Input: part model. Units: mm. Frame: model coordinates. Coordinates: 2 decimals unless noted, no trailing zeros. Loops run counter-clockwise (first coordinate to the right, second up) from the corner with the lowest first, then second, coordinate; pieces in that order, holes last.
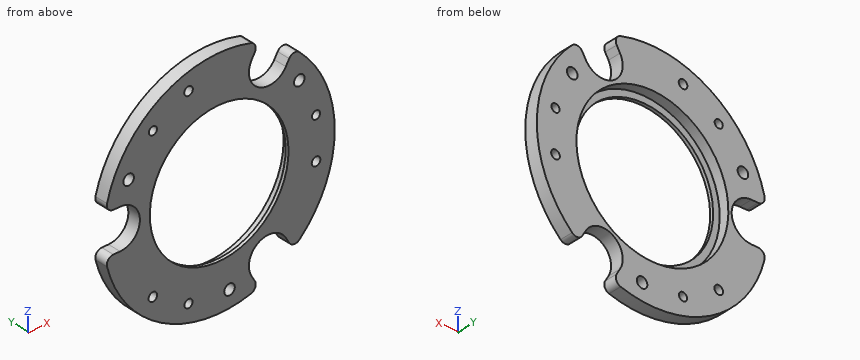
Autodesk Inventor part; units mm, degrees
ref_plane "YZ Plane" through (0, 0, 0) normal (1, 0, 0) x (0, 1, 0)
ref_plane "XZ Plane" through (0, 0, 0) normal (0, 1, 0) x (-1, 0, 0)
ref_plane "XY Plane" through (0, 0, 0) normal (0, 0, 1) x (1, 0, 0)
sketch "Sketch1" plane through (0, 0, 0) normal (1, 0, 0) x (0, 1, 0)
  line L0 (0, 35) -> (4, 35)
  line L1 (4, 35) -> (4, 23)
  line L2 (1, 21) -> (0, 21)
  line L3 (0, 21) -> (0, 35)
  line L4 (-0.8, 0) -> (4.8, 0)
  line L5 (1, 23) -> (1, 21)
  line L6 (4, 23) -> (1, 23)
  point P0 (0, 0)
  dimension "d0" = 21
  dimension "d2" = 35
  dimension "d51" = 4
  dimension "d52" = 3
  dimension "d53" = 23
revolve "Revolution1" add sketch "Sketch1" angle 360 about axis through (0, -10, 0) along (0, 1, 0)
sketch "Sketch2" plane through (0, 4, 0) normal (0, 1, 0) x (1, 0, 0)
  arc A0 (-30, -6) -> (-30, 6) centre (-30, 0) ccw
  line L0 (-30, -6) -> (-34.4819, -6)
  circle A1 centre (0, 0) radius 35
  line L1 (-30, 6) -> (-34.4819, 6)
  arc A2 (-34.4819, 6) -> (-34.4819, -6) centre (0, 0) ccw
  dimension "d6" = 12
  dimension "d7" = 30
extrude "Extrusion1" cut sketch "Sketch2" against normal blind 4 contours L0 A1 L1 A0 picked at (-31.3095, 0.2411)
pattern_circular "Circular Pattern1" count 3 over 360 about axis through (0, 0.5, 0) along (0, 1, 0) of "Extrusion1"
sketch "Sketch3" plane through (-34.4819, 4, -6) normal (0, 1, 0) x (1, 0, 0)
  point P0 (34.4819, -6)
sketch "Sketch4" plane through (-34.4819, 4, -6) normal (0, 1, 0) x (1, 0, 0)
  circle A0 centre (34.4819, -6) radius 30 construction
  arc A1 (4.4819, -12) -> (4.4819, 0) centre (4.4819, -6) ccw
  point P0 (7.0755, -18.2021)
  dimension "d13" = 60
  dimension "d14" = 24
hole "Hole1" at (-27.4064, 4, 12.2021) direction (0, -1, 0) diameter 3.2 end through all
pattern_circular "Circular Pattern2" count 3 over 360 about axis through (0, 0.5, 0) along (0, 1, 0) of "Hole1"
sketch "Sketch5" plane through (-34.4819, 4, -6) normal (0, 1, 0) x (1, 0, 0)
  circle A0 centre (34.4819, -6) radius 30 construction
  arc A1 (4.4819, -12) -> (4.4819, 0) centre (4.4819, -6) ccw
  point P0 (14.408, 16.2943)
  dimension "d25" = 60
  dimension "d26" = 48
hole "Hole2" at (-20.0739, 4, -22.2943) direction (0, -1, 0) diameter 2.6211 end through all
pattern_circular "Circular Pattern3" count 3 over 360 about axis through (0, 0.5, 0) along (0, 1, 0) of "Hole2"
sketch "Sketch6" plane through (-34.4819, 4, -6) normal (0, 1, 0) x (1, 0, 0)
  circle A0 centre (7.0755, -18.2021) radius 1.6
  line L0 (34.4819, -6) -> (7.0755, -18.2021) construction
  circle A1 centre (34.4819, -6) radius 21
  circle A2 centre (25.2114, -34.5317) radius 1.3106
  line L1 (34.4819, -6) -> (25.2114, -34.5317) construction
  circle A3 centre (34.4819, -6) radius 30 construction
  point P0 (14.408, -28.2943)
  dimension "d37" = 60
  dimension "d38" = 48
  dimension "d39" = 24
hole "Hole3" at (-20.0739, 4, 22.2943) direction (0, -1, 0) diameter 2.459 end through all
pattern_circular "Circular Pattern4" count 3 over 360 about axis through (0, 0.5, 0) along (0, 1, 0) of "Hole3"
fillet "Fillet1" radius 2 6 edges at (12.0448, 2, 32.8622) (22.4371, 2, 26.8622) (22.4371, 2, -26.8622) (12.0448, 2, -32.8622) (-34.4819, 2, -6) (-34.4819, 2, 6)
properties part number "MiddleRing-2023-1" material "Copper"
Item 1: Section query A-A (x = 0). Output: boundary loops of the cut face in (y, z), then the cut area to 3 significant figures.
Result:
outline: (0, -35) - (4, -35) - (4, -23) - (1, -23) - (1, -21) - (0, -21) - close; (0, 21) - (1, 21) - (1, 23) - (4, 23) - (4, 35) - (0, 35) - close
area: 100 mm2
Item 2: Section query D-D (z = 18). Output: boundary loops of the cut face in (x, y).
Result:
outline: (-30.02, 0) - (-10.82, 0) - (-10.82, 1) - (-14.32, 1) - (-14.32, 4) - (-30.02, 4) - close; (10.82, 0) - (22.71, 0) - (22.71, 4) - (14.32, 4) - (14.32, 1) - (10.82, 1) - close; (25.83, 0) - (30.02, 0) - (30.02, 4) - (25.83, 4) - close
Item 3: Section query C-C (x = -9). Output: boundary loops of the cut face in (y, z), then the cut area to 3 significant figures.
Result:
outline: (0, -33.82) - (4, -33.82) - (4, -29.73) - (0, -29.73) - close; (0, -27.33) - (4, -27.33) - (4, -21.17) - (1, -21.17) - (1, -18.97) - (0, -18.97) - close; (0, 18.97) - (1, 18.97) - (1, 21.17) - (4, 21.17) - (4, 27.25) - (0, 27.25) - close; (0, 29.81) - (4, 29.81) - (4, 33.82) - (0, 33.82) - close
area: 85.8 mm2
Item 4: Line query: L1, parallel to X at y = 3.25, z = -29; L2, parallel to Z at x = -26, y = 3.1; L3, parallel to Y at x = 22, z = 0.5. Output: solid intervals per line, ascending.
Result:
L1: x = -19.6 to -10.41, -8.13 to 1.77, 4.5 to 9.81
L2: z = -23.43 to -4.47, 4.47 to 11.44, 12.97 to 23.43
L3: y = 0 to 1
Item 5: Contact query for flat-ended pins moving along their axis: P1, Ø1, axis at y = 3.5, z = -23.5, coming from the -X side; P2, Ø1.5, axis at x = 5, y = 3, coming from the -Z side; P3, Ø1, axis at x = -30.5, y = 3, coming from the -Z side. Output: stop coordinate, or through.
Result:
P1: stops at x = -26.38
P2: stops at z = -34.74
P3: stops at z = -18.03
Item 6: Section query B-B (z = 0). Output: boundary loops of the cut face in (x, y), then the cut area to 3 significant figures.
Result:
outline: (-24, 0) - (-21, 0) - (-21, 1) - (-23, 1) - (-23, 4) - (-24, 4) - close; (21, 0) - (35, 0) - (35, 4) - (23, 4) - (23, 1) - (21, 1) - close
area: 56.0 mm2
